Could you check a few things on this model? Use its own coordinates, in mm. A direction names the side the tool comes from. Round coordinates to 2 decimals unless told otherwise and drop trailing zeros. Write each loop counter-clockwise with the first axis right and the second up, starting at its lowest first coordinate (ties: lowest second). Pieces come first, ordered by that corner, then holes. Notation, with made-up numbers: (33, -21) -> (47, -21) arc R26 cw to (47, 13) -> close; hole circle Ø7 at (57.5, 34.25). An arc over 180 degrees is marked (long way). Answer in a Markdown table with one row per item.
from build123d import *

# Parameters (mm, degrees)
SKETCH_1_W      = 70
SKETCH_1_H      = 10
EXTRUDE_1_DEPTH = 10
SKETCH_2_W      = 10
SKETCH_2_H      = 10
EXTRUDE_2_DEPTH = 42
EXTRUDE_3_DEPTH = 22


with BuildPart() as part:
    # 草图1 → 凸台-拉伸1 (new body)
    with BuildSketch(Plane(origin=(0, 0, 0), x_dir=(1, 0, 0), z_dir=(0, 1, 0))):
        with Locations((35, 5)):
            Rectangle(SKETCH_1_W, SKETCH_1_H)
    extrude(amount=EXTRUDE_1_DEPTH)

    # 草图2 → 凸台-拉伸2 (add)
    with BuildSketch(Plane.XY):
        with Locations((9.5, 5)):
            Rectangle(SKETCH_2_W, SKETCH_2_H)
        with Locations((60.5, 5)):
            Rectangle(SKETCH_2_W, SKETCH_2_H)
    extrude(amount=EXTRUDE_2_DEPTH)

    # 草图3 → 凸台-拉伸3 (add)
    with BuildSketch(Plane.XY.offset(42)):
        with BuildLine():
            Line((8.467001677, 0), (14.603921946, 0))
            ThreePointArc((14.603921946, 0), (35, -16), (55.396078054, 0))
            Line((55.396078054, 0), (61.532998323, 0))
            ThreePointArc((61.532998323, 0), (35, -22), (8.467001677, 0))
        make_face()
    extrude(amount=-EXTRUDE_3_DEPTH)


solid = part.part
1) Thinking about a two-plate mould opening in X: for faces 6 (the face through (4.5, 5, 21)), 7 (the face through (33, -17, 42)), 8 (the face through (35, 5, 0)), 9 (the face through (65.5, 5, 21)), which applies, +X half, -X half, draft (parallel to the pull), parting line (faces both ways), or undercut?
Findings:
| item | result |
|---|---|
| face 6 | -X half |
| face 7 | draft |
| face 8 | undercut |
| face 9 | +X half |
2) Imagine slicing it at D-D, the plane y = 8. Please give me the cut outline in (x, z).
Findings:
| item | result |
|---|---|
| outline | (0, -10) -> (70, -10) -> (70, 0) -> (65.5, 0) -> (65.5, 42) -> (55.5, 42) -> (55.5, 0) -> (14.5, 0) -> (14.5, 42) -> (4.5, 42) -> (4.5, 0) -> (0, 0) -> close |
3) For faces 1 (the face through (2, 5, 0)), 2 (the face through (68, 5, 0)), 3 (the face through (14.5, 5, 21)), 4 (the face through (35.523, -21.995, 31.154)), 5 (the face through (33, -17, 20)), which set-ups out of +Z, -Z, +X, -X, +Y, -Y let a thin tool reach every point of the face, with its end or its side?
Findings:
| item | result |
|---|---|
| face 1 | +Z, -X, +Y, -Y |
| face 2 | +Z, +X, +Y, -Y |
| face 3 | +Z, +Y |
| face 4 | +Z, -Z, -Y |
| face 5 | -Z, +X, -X, -Y |
4) For pin 1 (1 mm diameter, centred on x = 60, z = -4.5, fed in from -Y); pin 2 (11 mm diameter, centred on y = 7, z = 16, fed in from +X); pin 3 (8 mm diameter, centred on x = 50.5, y = -13, fed in from -Z); pin 4 (8 mm diameter, centred on y = -5.5, z = 15, fed in from -X), each with a flat end and sliding along its axis, tell me the tip position at first contact or that it passes through.
Findings:
| item | result |
|---|---|
| pin 1 | stops at y = 0 |
| pin 2 | stops at x = 65.5 |
| pin 3 | stops at z = 20 |
| pin 4 | passes through |
5) Imagine slicing it at C-C, the plane z = 26. Please give me the cut outline in (x, y), plus the area to 3 significant figures.
Findings:
| item | result |
|---|---|
| outline | (4.5, 0) -> (8.47, 0) arc R27 ccw to (61.53, 0) -> (65.5, 0) -> (65.5, 10) -> (55.5, 10) -> (55.5, 0) -> (55.4, 0) arc R21 cw to (14.6, 0) -> (14.5, 0) -> (14.5, 10) -> (4.5, 10) -> close |
| area | 592 mm^2 |
6) Imagine slicing it at A-A, the plane z = 1.5. Please give me the cut outline in (x, y).
Findings:
| item | result |
|---|---|
| outline | (4.5, 0) -> (14.5, 0) -> (14.5, 10) -> (4.5, 10) -> close; (55.5, 0) -> (65.5, 0) -> (65.5, 10) -> (55.5, 10) -> close |
7) Imagine slicing it at B-B, the plane x = 35. Please give me the cut outline in (y, z).
Findings:
| item | result |
|---|---|
| outline | (-22, 20) -> (-16, 20) -> (-16, 42) -> (-22, 42) -> close; (0, -10) -> (10, -10) -> (10, 0) -> (0, 0) -> close |
8) Please list where these lines run through material, in increasing order: line 1 (X direction, y = 8, z = 10); line 2 (Z direction, x = 22, y = -15.5); line 3 (Z direction, x = 27, y = 6.5).
Findings:
| item | result |
|---|---|
| line 1 | x = 4.5 to 14.5, 55.5 to 65.5 |
| line 2 | z = 20 to 42 |
| line 3 | z = -10 to 0 |
